from build123d import *

# Parameters (mm, degrees)
F0_R      = 2
F3_R      = 1
F4_DEPTH  = 2
F5_R      = 0.5
F6_R      = 2
F7_DEPTH  = 30
F8_W      = 2
F8_H      = 2
F9_DEPTH  = 50
F10_W     = 2
F10_H     = 1.97649955
F11_DEPTH = 25
F12_R     = 0.6
F13_DEPTH = 4.5506
F15_DEPTH = 10


with BuildPart() as f2:
    # F2: sweep along a path in F1
    with BuildLine(Plane.YZ) as f2_path:
        ThreePointArc((47.6558283438, -6.7940046368), (45.316272775, -0.3661285399), (39.3923101205, 3.0540728933))
        Line((39.3923101205, 3.0540728933), (5.8682408883, 8.9652708021))
        ThreePointArc((5.8682408883, 8.9652708021), (1.7860619516, 7.8714542526), (0, 4.041232037))
        Line((0, 4.041232037), (0, 0))
    # F0 (on Top) → F2 (sweep)
    with BuildSketch(Plane.XY):
        Circle(F0_R)
    sweep(path=f2_path.line)

    # F3 (on face) → F4 (cut)
    with BuildSketch(Plane(origin=(0, 0, -6.7940046368), x_dir=(1, 0, 0), z_dir=(0, 0, -1))):
        with Locations((0, -47.6558283438)):
            Circle(F3_R)
    extrude(amount=-F4_DEPTH, mode=Mode.SUBTRACT)

    # F5
    f5_edges = [f2.edges().sort_by_distance(p)[0] for p in [
        (-2, 47.655828, -6.794005),
    ]]
    fillet(f5_edges, radius=F5_R)

    # F6 (on face) → F7 (join)
    with BuildSketch(Plane(origin=(0, 0, 0), x_dir=(1, 0, 0), z_dir=(0, 0, -1))):
        Circle(F6_R)
    extrude(amount=F7_DEPTH)

    # F8 (on Front) → F9 (cut)
    with BuildSketch(Plane.XZ):
        with Locations((0.0787500758, -29.02350045)):
            Rectangle(F8_W, F8_H)
    extrude(amount=F9_DEPTH, mode=Mode.SUBTRACT)

    # F10 (on face) → F11 (cut)
    with BuildSketch(Plane.XZ):
        with Locations((0.0787500758, -29.011750225)):
            Rectangle(F10_W, F10_H)
    extrude(amount=-F11_DEPTH, mode=Mode.SUBTRACT)

    # F12 (on Right) → F13 (cut)
    with BuildSketch(Plane.YZ):
        with Locations((0, -29)):
            Circle(F12_R)
    extrude(amount=F13_DEPTH, mode=Mode.SUBTRACT)

    # F14 (on face) → F15 (cut)
    with BuildSketch(Plane.YZ.offset(-0.9212499242)):
        with BuildLine():
            ThreePointArc((0.6, -29), (0.4242640687, -28.5757359313), (0, -28.4))
            Line((0, -28.4), (0, -29.6))
            ThreePointArc((0, -29.6), (0.4242640687, -29.4242640687), (0.6, -29))
        make_face()
        with BuildLine():
            Line((0, -29.6), (0, -28.4))
            ThreePointArc((0, -28.4), (-0.6, -29), (0, -29.6))
        make_face()
    extrude(amount=-F15_DEPTH, mode=Mode.SUBTRACT)


solid = f2.part
Geometry check sheet. Reference: the model listing, model coordinates, mm. A direction names the side the tool comes from. Give positions to 0.01 mm unless a question says otherwise; leave off trailing zeros. Order: outer loops, then holes, each group sorted by start corner. A loop starts at its lowest first (then second) coordinate and runs counter-clockwise, first axis right, second up. Notation, with made-up numbers: M -16.5,85.25 L 32.5,85.25 A24 ccw 32.5,112.25 Z; hole C -6,21.25 d7. An arc over 180 degrees is marked long. Use a Markdown table: item, result.
Item 1: Tool access check on faces 4 (the flat face through (-1.3, 0, -30)), 5 (the flat face through (1.079, -1, -29)), 6 (the flat face through (0, 48, -4.794)). Record the directions out of +Z, -Z, +X, -X, +Y, -Y that give a thin tool (end or side, any length) a straight path to the whole face; none if there is none.
Answers follow:
| item | result |
|---|---|
| face 4 | -Z, +X, -X, +Y, -Y |
| face 5 | -Z, +Y, -Y |
| face 6 | -Z |
Item 2: Material ranges on line 1 along Y through (x, z) = (0, -5.8); line 2 along Y through (x, z) = (-0.1, -11); line 3 along Z through (x, y) = (1.5, 0), recorded low to high.
Answers follow:
| item | result |
|---|---|
| line 1 | y = -2 to 2, 45.59 to 46.66, 48.66 to 49.61 |
| line 2 | y = -2 to 2 |
| line 3 | z = -30 to -29.6, -28.4 to 7.91 |
Item 3: Depth check by flat-ended pin: P1, Ø1, axis at x = -1, y = 37, coming from the -Z side; P2, Ø1.5, axis at x = 0, z = -3, coming from the +Y side; P3, Ø0.6, axis at x = 0, y = 0, coming from the -Z side. Enter the tip coordinate at first touch or a pass-through.
Answers follow:
| item | result |
|---|---|
| P1 | stops at z = 1.48 |
| P2 | stops at y = 49.26 |
| P3 | stops at z = -28.02 |
Item 4: Section check A-A (z = -16). Record the cut outline in (x, y).
Answers follow:
| item | result |
|---|---|
| outline | C 0,0 d4 |
Item 5: Draft check along X on faces 1 (the flat face through (1, 47, -6.794)), 2 (the cylindrical face through (-0.22, 48.63, -5.81)), 3 (the cylindrical face through (-0.26, 22.74, 8.004)). Enter one of: +X half, -X half, draft (parallel to the pull), parting line (faces both ways), or undercut.
Answers follow:
| item | result |
|---|---|
| face 1 | draft |
| face 2 | undercut |
| face 3 | parting line |
